CAD build for the part. Positions are in the model's coordinates, mm. Coordinates: 2 decimals unless noted, no trailing zeros. Loops run counter-clockwise (first coordinate to the right, second up) from the corner with the lowest first, then second, coordinate; pieces in that order, holes last. Notation, with made-up numbers: (-0.5, -30) -> (44.5, -30) arc R23 ccw to (44.5, -3) -> close; hole circle Ø4 at (-24, -31). An arc over 180 degrees is marked (long way). Write item = value, one per line. Start each with the question number.
(1) Flat gauge pin, fed straight in: P1, Ø1.5, axis at y = 27, z = -71.5, coming from the +X side. Where does the tip first touch, or does it go through?
(2) Drill centre line: line 1 (Z direction, x = -2.25, y = 0). Where is it in solid material? Low to high. Write a range as from..to.
(3) Band-saw the part on A-A (y = 0). Write the cut outline in (x, z), and give its area (3 significant figures).
(4) Pull direction Y, two halves, no side cores. Call faces 1 (the face through (0, -1, -2)), 2 (the face through (-3, -76.2, 2)), 3 (the face through (-3.131, -0.982, -89.844)): +Y half, -Y half, draft (parallel to the pull), parting line (faces both ways), or undercut.
```python
from build123d import *

# Parameters (mm, degrees)
F1_DEPTH = 76.2
F2_R     = 4.5318999151
F3_DEPTH = 6.351


# Not quite as in the source:
# - a feature names something its author has since deleted; it is built from what else it names


with BuildPart() as f1:
    # F0 (on Front) → F1 (new body, symmetric)
    with BuildSketch(Plane.XZ):
        Polygon((0, -127), (0, 0), (0, 127), (-6.35, 127), (-6.35, 0), (-6.35, -127), align=None)
    extrude(amount=F1_DEPTH, both=True)

    # F2 (on face) → F3 (cut, through all)
    with BuildSketch(Plane.YZ):
        with Locations((0, -85.4202)):
            Circle(F2_R)
        with Locations((0, 85.4202)):
            Circle(F2_R)
    extrude(amount=-F3_DEPTH, mode=Mode.SUBTRACT)


solid = f1.part
```
Findings below:
q1.P1 = 0
q2.line_1 = -127..-89.95, -80.89..80.89, 89.95..127
q3.outline = (-6.35, -127) -> (0, -127) -> (0, -89.95) -> (-6.35, -89.95) -> close; (-6.35, -80.89) -> (0, -80.89) -> (0, 80.89) -> (-6.35, 80.89) -> close; (-6.35, 89.95) -> (0, 89.95) -> (0, 127) -> (-6.35, 127) -> close
q3.area = 1,500 mm²
q4.face_1 = draft
q4.face_2 = -Y half
q4.face_3 = undercut
